```python
from build123d import *

# Parameters (mm, degrees)
BOSS_EXTRUDE1_DEPTH = 76.2
CUT_EXTRUDE1_DEPTH  = 10
SKETCH4_R           = 3.5
CUT_EXTRUDE2_DEPTH  = 10


with BuildPart() as part:
    # Sketch2 → Boss-Extrude1 (new, symmetric)
    with BuildSketch(Plane.XY):
        with BuildLine():
            Line((-38.1, 0), (38.1, 0))
            Line((38.1, 0), (38.1, 101.6))
            Line((38.1, 101.6), (34.925, 101.6))
            ThreePointArc((34.925, 101.6), (32.67993597, 100.67006403), (31.75, 98.425))
            Line((31.75, 98.425), (31.75, 9.525))
            ThreePointArc((31.75, 9.525), (30.82006403, 7.27993597), (28.575, 6.35))
            Line((28.575, 6.35), (-34.925, 6.35))
            ThreePointArc((-34.925, 6.35), (-37.17006403, 5.42006403), (-38.1, 3.175))
            Line((-38.1, 3.175), (-38.1, 0))
        make_face()
    extrude(amount=BOSS_EXTRUDE1_DEPTH, both=True)

    # Sketch3 → Cut-Extrude1 (cut)
    with BuildSketch(Plane(origin=(38.1, 0, 0), x_dir=(0, 0, -1), z_dir=(1, 0, 0))):
        with BuildLine():
            Line((-28.25, 76.2), (-28.25, 25.4))
            ThreePointArc((-28.25, 25.4), (-31.75, 21.9), (-35.25, 25.4))
            Line((-35.25, 25.4), (-35.25, 76.2))
            ThreePointArc((-35.25, 76.2), (-31.75, 79.7), (-28.25, 76.2))
        make_face()
        with BuildLine():
            Line((28.25, 76.2), (28.25, 25.4))
            ThreePointArc((28.25, 25.4), (31.75, 21.9), (35.25, 25.4))
            Line((35.25, 25.4), (35.25, 76.2))
            ThreePointArc((35.25, 76.2), (31.75, 79.7), (28.25, 76.2))
        make_face()
        with BuildLine():
            Line((3.5, 76.2), (3.5, 25.4))
            ThreePointArc((3.5, 25.4), (0, 21.9), (-3.5, 25.4))
            Line((-3.5, 25.4), (-3.5, 76.2))
            ThreePointArc((-3.5, 76.2), (0, 79.7), (3.5, 76.2))
        make_face()
    extrude(amount=-CUT_EXTRUDE1_DEPTH, mode=Mode.SUBTRACT)

    # Sketch4 → Cut-Extrude2 (cut)
    with BuildSketch(Plane.XZ):
        with Locations(Location((0, 25.4, 0), (0, 0, 270))):
            Circle(SKETCH4_R)
        with Locations((0, -25.4)):
            Circle(SKETCH4_R)
        with Locations(Location((0, 0, 0), (0, 0, 270))):
            Circle(SKETCH4_R)
    extrude(amount=-CUT_EXTRUDE2_DEPTH, mode=Mode.SUBTRACT)


solid = part.part
```
Input: part model. Units: mm. Frame: model coordinates. A direction names the side the tool comes from. Give positions to 0.01 mm unless a question says otherwise; leave off trailing zeros. Loops run counter-clockwise (first coordinate to the right, second up) from the corner with the lowest first, then second, coordinate; pieces in that order, holes last.
1) Section query C-C on y = 69. Return the cut outline in (x, z), and give its area (3 significant figures).
A:
outline: (31.75, -76.2) - (38.1, -76.2) - (38.1, -35.25) - (31.75, -35.25) - close; (31.75, -28.25) - (38.1, -28.25) - (38.1, -3.5) - (31.75, -3.5) - close; (31.75, 3.5) - (38.1, 3.5) - (38.1, 28.25) - (31.75, 28.25) - close; (31.75, 35.25) - (38.1, 35.25) - (38.1, 76.2) - (31.75, 76.2) - close
area: 834 mm2
2) Mould query, pull axis Y, two halves, no side actions, for faces 3 (the cylindrical face through (35, 21.9, -0.1)), 4 (the flat face through (8, 0, 1)), 5 (the cylindrical face through (1.05, 3.13, 22.06)). Classes: released by +Y, released by -Y, zero draft, split by the parting line, or undercut.
A:
face 3: undercut
face 4: released by -Y
face 5: zero draft
3) Section query B-B on z = 0. Return the cut outline in (x, y) (3 decimals).
A:
outline: (-38.1, 0) - (-3.5, 0) - (-3.5, 6.35) - (-34.925, 6.35) arc R3.175 ccw to (-38.1, 3.175) - close; (3.5, 0) - (38.1, 0) - (38.1, 21.9) - (31.75, 21.9) - (31.75, 9.525) arc R3.175 cw to (28.575, 6.35) - (3.5, 6.35) - close; (31.75, 79.7) - (38.1, 79.7) - (38.1, 101.6) - (34.925, 101.6) arc R3.175 ccw to (31.75, 98.425) - close
4) Reachability of faces 1 (the cylindrical face through (-3.417, 3.131, 0.759)), 2 (the flat face through (35, 51, -3.5)) from +Z, -Z, +X, -X, +Y, -Y: full face, straight path, thin tool, end or side. Return the list, or none.
A:
face 1: +Y, -Y
face 2: +X, -X
5) Line query: L1, parallel to X at y = 3, z = -25; L2, parallel to X at y = 67, z = -17.5; L3, parallel to Y at x = 20.5, z = 54.5. Output: solid intervals per line, ascending.
A:
L1: x = -38.1 to -3.48, 3.48 to 38.1
L2: x = 31.75 to 38.1
L3: y = 0 to 6.35
6) Section query A-A on z = -25.4. Return the cut outline in (x, y) (3 decimals).
A:
outline: (-38.1, 0) - (-3.5, 0) - (-3.5, 6.35) - (-34.925, 6.35) arc R3.175 ccw to (-38.1, 3.175) - close; (3.5, 0) - (38.1, 0) - (38.1, 101.6) - (34.925, 101.6) arc R3.175 ccw to (31.75, 98.425) - (31.75, 9.525) arc R3.175 cw to (28.575, 6.35) - (3.5, 6.35) - close
7) Contact query for flat-ended pins moving along their axis: pin 1 (8 mm diameter, centred on y = 38, z = 29, fed in from -X); pin 2 (8 mm diameter, centred on x = 0, z = 25.4, fed in from -Y); pin 3 (6 mm diameter, centred on x = -1.5, z = -52, fed in from +Y). Output: stop coordinate, or through.
A:
pin 1: stops at x = 31.75
pin 2: stops at y = 0
pin 3: stops at y = 6.35
8) Section query D-D on x = 0. Return the cut outline in (y, z).
A:
outline: (0, -76.2) - (6.35, -76.2) - (6.35, -28.9) - (0, -28.9) - close; (0, -21.9) - (6.35, -21.9) - (6.35, -3.5) - (0, -3.5) - close; (0, 3.5) - (6.35, 3.5) - (6.35, 21.9) - (0, 21.9) - close; (0, 28.9) - (6.35, 28.9) - (6.35, 76.2) - (0, 76.2) - close
